The listing builds one solid part. Answer for the finished solid, in the listing's coordinates (mm). Face numbers are marked on the shaded views. A direction names the side the tool comes from. Coordinates: 2 decimals unless noted, no trailing zeros. Order: outer loops, then holes, each group sorted by start corner. A loop starts at its lowest first (then second) coordinate and runs counter-clockwise, first axis right, second up. Notation, with made-up numbers: (37.5, 66) -> (76.5, 66) arc R21 cw to (76.5, 78) -> close; hole circle Ø11 at (-35.5, 32). An arc over 180 degrees is marked (long way). Return JSON: item names as keys, results as strings.
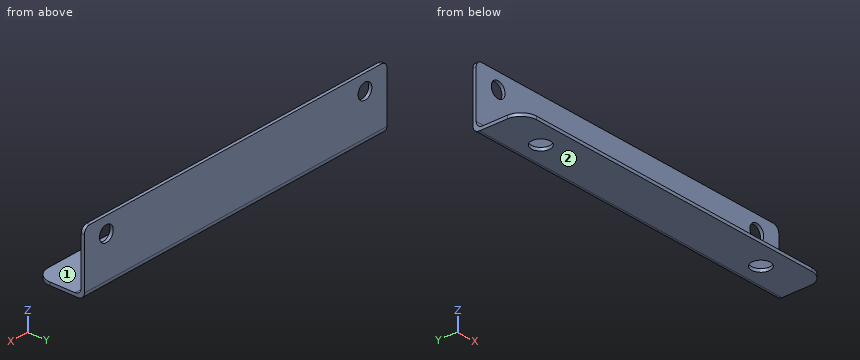
from build123d import *

# Parameters (mm, degrees)
SKETCH1_R           = 3
BOSS_EXTRUDE1_DEPTH = 1
SKETCH2_W           = 110
SKETCH2_H           = 20
SKETCH2_R           = 2.5
BOSS_EXTRUDE2_DEPTH = 1
FILLET1_R           = 2


with BuildPart() as part:
    # Sketch1 → Boss-Extrude1 (new body)
    with BuildSketch(Plane.XY):
        with BuildLine():
            Line((-55, 0), (55, 0))
            Line((55, 0), (55, -10))
            ThreePointArc((55, -10), (53.535533906, -13.535533906), (50, -15))
            Line((50, -15), (-50, -15))
            ThreePointArc((-50, -15), (-53.535533906, -13.535533906), (-55, -10))
            Line((-55, -10), (-55, 0))
        make_face()
        with Locations((40, -7.5)):
            Circle(SKETCH1_R, mode=Mode.SUBTRACT)
        with Locations(Location((-40, -7.5, 0), (0, 0, 180))):
            Circle(SKETCH1_R, mode=Mode.SUBTRACT)
    extrude(amount=BOSS_EXTRUDE1_DEPTH)

    # Sketch2 → Boss-Extrude2 (add)
    with BuildSketch(Plane(origin=(0, 0, 0), x_dir=(1, 0, 0), z_dir=(0, 1, 0))):
        with Locations((0, -10)):
            Rectangle(SKETCH2_W, SKETCH2_H)
        with Locations(Location((47, -15, 0), (0, 0, 270))):
            Circle(SKETCH2_R, mode=Mode.SUBTRACT)
        with Locations(Location((-47, -15, 0), (0, 0, 90))):
            Circle(SKETCH2_R, mode=Mode.SUBTRACT)
    extrude(amount=BOSS_EXTRUDE2_DEPTH)

    # Fillet1
    fillet1_edges = [part.edges().sort_by_distance(p)[0] for p in [
        (0, 0, 1),
        (0, 1, 0),
        (55, 0.5, 20),
        (-55, 0.5, 20),
    ]]
    fillet(fillet1_edges, radius=FILLET1_R)


solid = part.part
1. The part is cut by section C-C on x = 27.5. Give the vertices of the cut face in (y, z), and give its area (3 significant figures).
Answer block:
{"outline": "(-15, 0) -> (-1, 0) arc R2 ccw to (1, 2) -> (1, 20) -> (0, 20) -> (0, 3) arc R2 cw to (-2, 1) -> (-15, 1) -> close", "area": "35.0 mm2"}
2. Consider line 1 (X direction, y = 0.6, z = 15); line 2 (Z direction, x = -34.5, y = -12.25). Determine where each line is inside the solid, lowest interval first. Write a range as from..to.
Answer block:
{"line 1": "x = -55..-49.5, -44.5..44.5, 49.5..55", "line 2": "z = 0..1"}
3. The part is cut by section A-A on x = 40. Give the vertices of the cut face in (y, z), and give its area (3 significant figures).
Answer block:
{"outline": "(-15, 0) -> (-10.5, 0) -> (-10.5, 1) -> (-15, 1) -> close; (-4.5, 0) -> (-1, 0) arc R2 ccw to (1, 2) -> (1, 20) -> (0, 20) -> (0, 3) arc R2 cw to (-2, 1) -> (-4.5, 1) -> close", "area": "29.0 mm2"}
4. The part is cut by section D-D on x = -47. Give the vertices of the cut face in (y, z), and give its area (3 significant figures).
Answer block:
{"outline": "(-15, 0) -> (-1, 0) arc R2 ccw to (1, 2) -> (1, 12.5) -> (0, 12.5) -> (0, 3) arc R2 cw to (-2, 1) -> (-15, 1) -> close; (0, 17.5) -> (1, 17.5) -> (1, 20) -> (0, 20) -> close", "area": "30.0 mm2"}
5. For the marked faces 1 and 2, determine the directions among +Z, -Z, +X, -X, +Y, -Y from which every point of the face is accessible in a straight line to the end or side of a thin tool.
Answer block:
{"face 1": "+Z, +X, -X, -Y", "face 2": "-Z, +X, -X, +Y, -Y"}
6. The part is cut by section B-B on z = 15. Give the vertices of the cut face in (x, y).
Answer block:
{"outline": "(-55, 0) -> (-49.5, 0) -> (-49.5, 1) -> (-55, 1) -> close; (-44.5, 0) -> (44.5, 0) -> (44.5, 1) -> (-44.5, 1) -> close; (49.5, 0) -> (55, 0) -> (55, 1) -> (49.5, 1) -> close"}
7. Each of these flat-tipped pins is pushed along its axis until it touches: pin 1 Ø6 at (x, z) = (-47, 15) entering from -Y; pin 2 Ø5.5 at (x, y) = (-40, -7.5) entering from +Z; pin 3 Ø8 at (x, y) = (40, -7.5) entering from +Z. Where does it stop, or does it pass through?
Answer block:
{"pin 1": "stops at y = 0", "pin 2": "passes through", "pin 3": "stops at z = 1"}
